The drawing under review shows one solid part. Ordinate dimensions are in mm from its lowest x, y, z. A direction names the side the tool comes from. Round coordinates to 2 decimals unless told otherwise and drop trailing zeros. Order: outer loops, then holes, each group sorted by start corner. A loop starts at its lowest first (then second) coordinate and runs counter-clockwise, first axis right, second up. Notation, with made-up numbers: M -28.5,78.5 L 10.5,78.5 A32 cw 10.5,109.5 Z; hole C 42,2 d11. An arc over 180 degrees is marked long. Answer as a JSON object with one key per item and string values. Group by question number.
1. Add section A-A on z = 7.25. State the section outline as (x, y) points, and give its area (3 significant figures).
2. Machinability: for the marked faces 4 and 5, which of the approach directions +Z, -Z, +X, -X, +Y, -Y give a long, thin tool a straight path to every point of the face, cutting with its end or side? Answer none if there is none.
3. Clearance check with a flat-ended pin moving along its axis: P1, Ø3, axis at y = 3, z = 9.5, coming from the +X side. State where the tip first meets the part, or that it passes through.
4. Add section D-D on x = 1. State the section outline as (y, z) points, and give its area (3 significant figures).
5. Mouldability with a two-part tool opening along Y and no side actions: class the marked faces 1, 2 and 3 as released by +Y, released by -Y, zero draft, split by the parting line, or undercut.
6. Add section C-C on y = 0.85. State the section outline as (x, z) points.
7. To check wall thickness, follow probe 1 along Z at (x, y) = (2.75, 4.65); probe 2 along X at (y, z) = (3.9, 8) (1 decimal); probe 3 along Y at (x, z) = (4.75, 2.5) (1 decimal). State the ranges of each line that lie inside material, in increasing order. Write a range as [from, to].
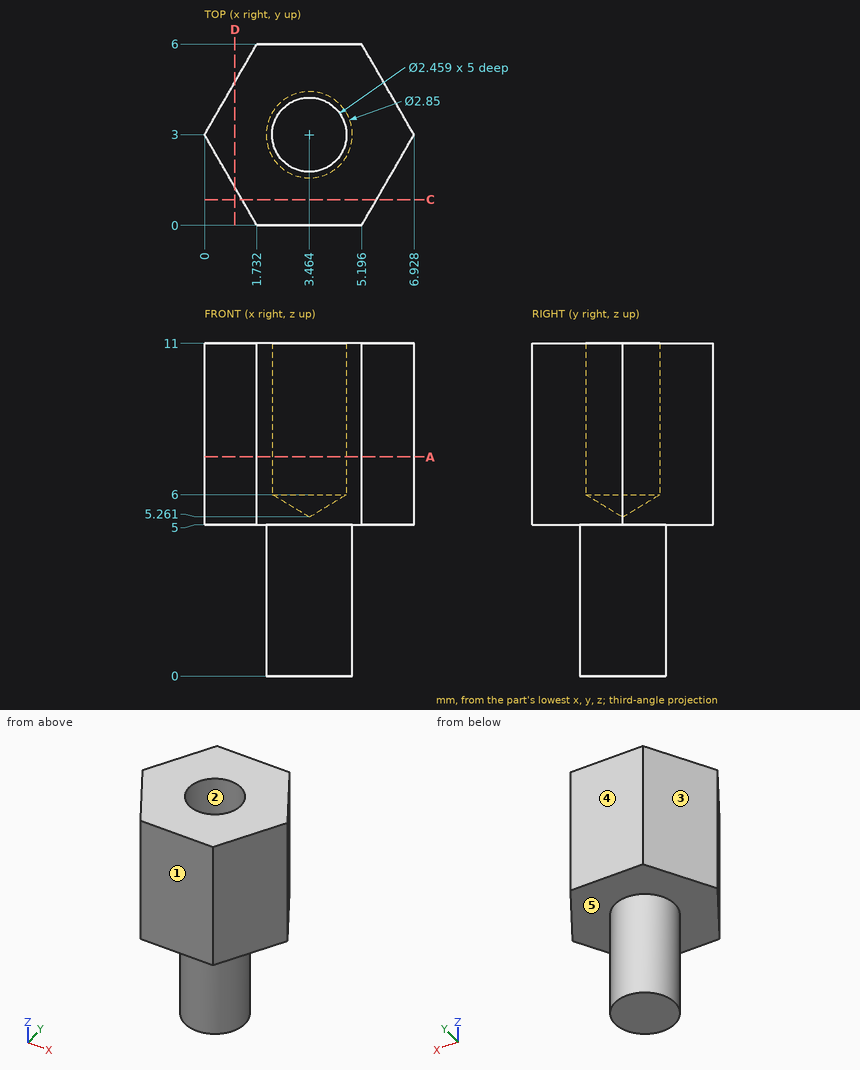
Recorded:
{
 "1": {"outline": "M 0,3 L 1.73,0 L 5.2,0 L 6.93,3 L 5.2,6 L 1.73,6 Z; hole C 3.46,3 d2.46", "area": "26.4 mm²"},
 "2": {"face 4": "+Z, -Z, +X, -X, +Y", "face 5": "-Z"},
 "3": {"P1": "stops at x = 6.93"},
 "4": {"outline": "M 1.27,5 L 4.73,5 L 4.73,11 L 1.27,11 Z", "area": "20.8 mm²"},
 "5": {"face 1": "released by -Y", "face 2": "undercut", "face 3": "released by +Y"},
 "6": {"outline": "M 1.24,5 L 5.69,5 L 5.69,11 L 1.24,11 Z"},
 "7": {"probe 1": "z = [5, 11]", "probe 2": "x = [0.5, 2.6], [4.3, 6.4]", "probe 3": "y = [2.4, 3.6]"}
}
